For this review, take the finished solid that the model builds, in its own axes (mm). A direction names the side the tool comes from. Round coordinates to 2 decimals unless told otherwise and drop trailing zeros. Order: outer loops, then holes, each group sorted by start corner. A loop starts at its lowest first (then second) coordinate and runs counter-clockwise, first axis right, second up. Notation, with made-up numbers: M -8,66 L 23,66 A23 cw 23,90 Z; hole C 86,88 d2. An arc over 180 degrees is marked long. Answer as a JSON object with one key per item and string values.
from build123d import *
from build123d.topology import SkipClean

# Parameters (mm, degrees)
SHELL1_T                 = 4
SKETCH4_W                = 50
SKETCH4_H                = 20
BOSS_EXTRUDE1_DEPTH      = 4
BOSS_EXTRUDE2_DEPTH      = 10.049697
BOSS_EXTRUDE2_DEPTH_BACK = 9.950303
SKETCH7_W                = 4
SKETCH7_H                = 20
SKETCH8_W                = 20
SKETCH8_H                = 4
BOSS_EXTRUDE3_DEPTH      = 47


with BuildPart() as part:
    # Boundary1: read off the stored shape, not the designer's step
    # Boundary1: loft between two sections, ruled curve by curve
    boundary1_from = [
        Edge.make_line((-15, 0, 15), (15, 0, 15)),
        Edge.make_line((15, 0, 15), (15, 0, -15)),
        Edge.make_line((15, 0, -15), (-15, 0, -15)),
        Edge.make_line((-15, 0, -15), (-15, 0, 15)),
    ]
    boundary1_to = [
        Edge.make_line((-66, 50, 37.5), (66, 50, 37.5)),
        Edge.make_line((66, 50, 37.5), (66, 50, -37.5)),
        Edge.make_line((66, 50, -37.5), (-66, 50, -37.5)),
        Edge.make_line((-66, 50, -37.5), (-66, 50, 37.5)),
    ]
    boundary1 = Solid(Shell([*[Face.make_surface_from_curves(boundary1_from[k], boundary1_to[k]) for k in range(4)], Face(Wire(boundary1_from)), Face(Wire(boundary1_to))]))
    add(boundary1)

    # Shell1
    shell1_openings = [part.faces().sort_by_distance(p)[0] for p in [
        (0, 0, 0),
        (0, 50, 0),
    ]]
    offset(amount=SHELL1_T, openings=shell1_openings, kind=Kind.INTERSECTION)

    # Sketch4 → Boss-Extrude1 (add)
    with BuildSketch(Plane(origin=(-10.15178535, -10.354821057, 0), x_dir=(0.7140728391445788, -0.7000714109260574, 0), z_dir=(-0.7000714109260574, -0.7140728391445788, 0))):
        with Locations((-39.791092587, 0.049697146)):
            Rectangle(SKETCH4_W, SKETCH4_H)
    extrude(amount=BOSS_EXTRUDE1_DEPTH)

    # Sketch7 → Boss-Extrude2 (add, two sides: drawn at the far end of the back side and taken through both)
    with SkipClean():  # the faces are left unmerged after this step: merging them gives an invalid solid
        with BuildSketch(Plane.XY.offset(-BOSS_EXTRUDE2_DEPTH_BACK)):
            with Locations((-22.713702827, -10)):
                Rectangle(SKETCH7_W, SKETCH7_H)
        extrude(amount=BOSS_EXTRUDE2_DEPTH + BOSS_EXTRUDE2_DEPTH_BACK)

    # Sketch8 → Boss-Extrude3 (add)
    with SkipClean():  # the faces are left unmerged after this step: merging them gives an invalid solid
        with BuildSketch(Plane.ZY.offset(24.713702827)):
            with Locations((0.049697146, -18)):
                Rectangle(SKETCH8_W, SKETCH8_H)
        extrude(amount=BOSS_EXTRUDE3_DEPTH)


solid = part.part
1) For L1, parallel to Z at x = 42.5, y = 33; L2, parallel to Z at x = 28.5, y = 31.5 (3 decimals); L3, parallel to X at y = 44.5, z = -8.5, list the stretches that pass through material, from the lowest coordinate up.
Geometry check:
{"L1": "z = -34.24 to -29.85, 29.85 to 34.24", "L2": "z = -33.561 to -29.175, 29.175 to 33.561", "L3": "x = -66.1 to -60.39, 60.39 to 66.1"}
2) Machinability: for faces 1 (the flat face through (-20.714, -10, 0)), 2 (the flat face through (-48, -16, 0)), 3 (the flat face through (-57.904, 36.461, -0.586)), which of the approach directions +Z, -Z, +X, -X, +Y, -Y give a long, thin tool a straight path to every point of the face, cutting with its end or side? Answer none if there is none.
Geometry check:
{"face 1": "+Z, -Z, +X, -Y", "face 2": "+Z, -Z, -X", "face 3": "-X"}
3) Add section A-A on y = -10.5. State the section outline as (x, z) points.
Geometry check:
{"outline": "M -24.71,-9.95 L -20.71,-9.95 L -20.71,10.05 L -24.71,10.05 Z"}
4) Mouldability with a two-part tool opening along Y and no side actions: class faces 4 (the flat face through (-1.004, 30.906, 33.294)), 5 (the flat face through (-42.207, 15.47, 0.19)), 6 (the flat face through (-71.714, -18, 0)) as +Y half, -Y half, draft (parallel to the pull), parting line (faces both ways), or undercut.
Geometry check:
{"face 4": "-Y half", "face 5": "undercut", "face 6": "draft"}
5) Insertion check: P1, Ø5, axis at x = 29.5, z = -32.5, coming from the -Y side; P2, Ø6, axis at x = -46.5, y = 35.5, coming from the -Z side; P3, Ø19.5, axis at x = 0, z = -0.5, coming from the -Y side; P4, Ø11.5, axis at x = -42, y = 15.5, coming from the +Z side. Each pin has a flat end and moves straight along its axis. Give the tip position at first contact, or say it passes through.
Geometry check:
{"P1": "stops at y = 23.59", "P2": "stops at z = -36.71", "P3": "passes through", "P4": "stops at z = 28.95"}
